Could you check a few things on this model? Use its own coordinates, in mm. Give positions to 0.01 mm unless a question says otherwise; leave off trailing zeros. Loops run counter-clockwise (first coordinate to the right, second up) from the corner with the lowest first, then second, coordinate; pieces in that order, holes last. Notation, with made-up numbers: M 7.25,12.25 L 60.25,12.25 A26 cw 60.25,50.25 Z; hole C 2,74 d5. An arc over 180 degrees is marked long. Return JSON: item names as keys, results as strings. Group by question number.
1. Please list where these lines run through material, in increasing order: line 1 (X direction, y = -11.5, z = 0.6); line 2 (X direction, y = 25.5, z = 0.9).
2. If we section it at A-A (x = 8.5): Write out the boundary of the cut face in (y, z), plus the area to 3 significant figures.
3. If we section it at D-D (z = 2): Write out the boundary of the cut face in (x, y).
4. If we section it at C-C (x = -27): Write out the boundary of the cut face in (y, z), plus the area to 3 significant figures.
5. For pin 1 (8 mm diameter, centred on x = -26, y = -10.5, fed in from -Z), with a flat end and sliding along its axis, tell me the tip position at first contact or that it passes through.
Autodesk Inventor part; units mm, degrees
ref_plane "YZ Plane" through (0, 0, 0) normal (1, 0, 0) x (0, 1, 0)
ref_plane "XZ Plane" through (0, 0, 0) normal (0, 1, 0) x (-1, 0, 0)
ref_plane "XY Plane" through (0, 0, 0) normal (0, 0, 1) x (1, 0, 0)
sketch "Sketch1" plane through (0, 0, 0) normal (0, 0, 1) x (1, 0, 0)
  line L0 (-37.1, -37.1) -> (37.1, -37.1)
  line L1 (37.1, -37.1) -> (37.1, 37.1)
  line L2 (37.1, 37.1) -> (-37.1, 37.1)
  line L3 (-37.1, 37.1) -> (-37.1, -37.1)
  line L4 (-37.1, -37.1) -> (37.1, 37.1) construction
  line L5 (37.1, -37.1) -> (-37.1, 37.1) construction
  line L6 (15.1, -15.1) -> (-15.1, -15.1)
  line L7 (-15.1, -15.1) -> (-15.1, 15.1)
  line L8 (-15.1, 15.1) -> (15.1, 15.1)
  line L9 (15.1, 15.1) -> (15.1, -15.1)
  line L10 (15.1, -15.1) -> (-15.1, 15.1) construction
  line L11 (-15.1, -15.1) -> (15.1, 15.1) construction
  point P0 (0, 0)
  dimension "d172" = 30.2
  dimension "d181" = 22
  dimension "d187" = 22
extrude "Plate5" add sketch "Sketch1" along normal blind 3
sketch "Sketch9" plane through (0, 0, 3) normal (0, 0, 1) x (1, 0, 0)
  circle A0 centre (26.5165, -26.5165) radius 2.75
  line L0 (26.5165, 26.5165) -> (-26.5165, 26.5165) construction
  line L1 (-26.5165, 26.5165) -> (-26.5165, -26.5165) construction
  line L2 (-26.5165, -26.5165) -> (26.5165, -26.5165) construction
  line L3 (26.5165, -26.5165) -> (26.5165, 26.5165) construction
  line L4 (26.5165, 26.5165) -> (-26.5165, -26.5165) construction
  line L5 (-26.5165, 26.5165) -> (26.5165, -26.5165) construction
  circle A1 centre (-26.5165, -26.5165) radius 2.75
  circle A2 centre (26.5165, 26.5165) radius 2.75
  circle A3 centre (-26.5165, 26.5165) radius 2.75
  circle A4 centre (0, 0) radius 37.5 construction
  line L6 (-15.1, -15.1) -> (-15.1, 15.1)
  line L7 (-15.1, 15.1) -> (15.1, 15.1)
  line L8 (15.1, 15.1) -> (15.1, -15.1)
  line L9 (15.1, -15.1) -> (-15.1, -15.1)
  line L10 (37.1, -37.1) -> (-37.1, -37.1)
  line L11 (37.1, 37.1) -> (37.1, -37.1)
  line L12 (-37.1, 37.1) -> (37.1, 37.1)
  line L13 (-37.1, -37.1) -> (-37.1, 37.1)
  line L14 (-15, 15) -> (15, 15) construction
  line L15 (15, 15) -> (15, -15) construction
  line L16 (15, -15) -> (-15, -15) construction
  line L17 (-15, -15) -> (-15, 15) construction
  line L18 (-15, -15) -> (15, 15) construction
  dimension "d188" = 75
  dimension "d174" = 5.5
  dimension "d184" = 30
  dimension "d185" = 30
  dimension "d186" = 16.2868
extrude "Cut2" cut sketch "Sketch9" against normal blind 3 contours A0 | A1 | A2 | A3
fillet "Corner Round1" radius 6 4 edges at (37.1, 37.1, 1.5) (-37.1, 37.1, 1.5) (-37.1, -37.1, 1.5) (37.1, -37.1, 1.5)
fillet "Corner Round2" radius 1 4 edges at (-15.1, 15.1, 1.5) (-15.1, -15.1, 1.5) (15.1, -15.1, 1.5) (15.1, 15.1, 1.5)
properties part number "ANP 1425 FDS Way FLANGE" material "Stainless Steel"
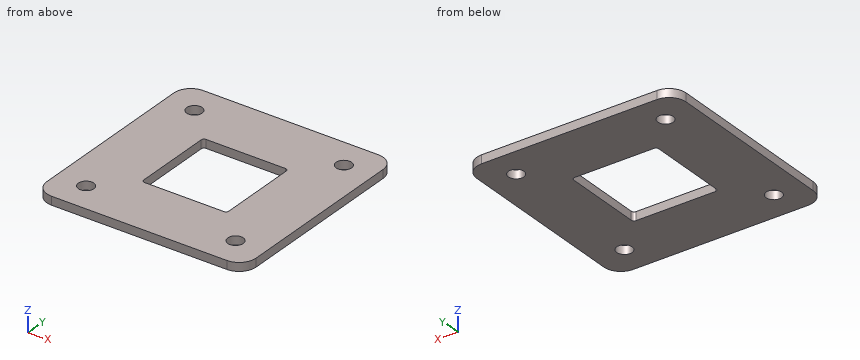
Answer:
{
 "1": {"line 1": "x = -37.1 to -15.1, 15.1 to 37.1", "line 2": "x = -37.1 to -29.07, -23.96 to 23.96, 29.07 to 37.1"},
 "2": {"outline": "M -37.1,0 L -15.1,0 L -15.1,3 L -37.1,3 Z; M 15.1,0 L 37.1,0 L 37.1,3 L 15.1,3 Z", "area": "132 mm²"},
 "3": {"outline": "M -37.1,-31.1 A6 ccw -31.1,-37.1 L 31.1,-37.1 A6 ccw 37.1,-31.1 L 37.1,31.1 A6 ccw 31.1,37.1 L -31.1,37.1 A6 ccw -37.1,31.1 Z; hole C -26.52,-26.52 d5.5; hole C -26.52,26.52 d5.5; hole M -15.1,-14.1 A1 ccw -14.1,-15.1 L 14.1,-15.1 A1 ccw 15.1,-14.1 L 15.1,14.1 A1 ccw 14.1,15.1 L -14.1,15.1 A1 ccw -15.1,14.1 Z; hole C 26.52,-26.52 d5.5; hole C 26.52,26.52 d5.5"},
 "4": {"outline": "M -37.1,0 L -29.22,0 L -29.22,3 L -37.1,3 Z; M -23.81,0 L 23.81,0 L 23.81,3 L -23.81,3 Z; M 29.22,0 L 37.1,0 L 37.1,3 L 29.22,3 Z", "area": "190 mm²"},
 "5": {"pin 1": "stops at z = 0"}
}
